from build123d import *

# Parameters (mm, degrees)
IZIM1_W                     = 30
IZIM1_H                     = 30
IZIM1_R                     = 4.75
Y_KSEKLIK_EKSTR_ZYON1_DEPTH = 5
IZIM2_R                     = 10
IZIM2_R_2                   = 4.75
Y_KSEKLIK_EKSTR_ZYON2_DEPTH = 20
IZIM3_R                     = 1.5
KES_EKSTR_ZYON1_DEPTH       = 7


with BuildPart() as part:
    # Çizim1 → Yükseklik-Ekstrüzyon1 (new body)
    with BuildSketch(Plane(origin=(0, 0, 0), x_dir=(1, 0, 0), z_dir=(0, 1, 0))):
        with Locations((15, 15)):
            Rectangle(IZIM1_W, IZIM1_H)
        with Locations(Location((15, 15, 0), (0, 0, 270))):
            Circle(IZIM1_R, mode=Mode.SUBTRACT)
    extrude(amount=Y_KSEKLIK_EKSTR_ZYON1_DEPTH)

    # Çizim2 → Yükseklik-Ekstrüzyon2 (add)
    with BuildSketch(Plane(origin=(0, 5, 0), x_dir=(1, 0, 0), z_dir=(0, 1, 0))):
        with Locations(Location((15, 15, 0), (0, 0, 90))):
            Circle(IZIM2_R)
        with Locations(Location((15, 15, 0), (0, 0, 270))):
            Circle(IZIM2_R_2, mode=Mode.SUBTRACT)
    extrude(amount=Y_KSEKLIK_EKSTR_ZYON2_DEPTH)

    # Çizim3 → Kes-Ekstrüzyon1 (cut)
    with BuildSketch(Plane(origin=(0, 5, 0), x_dir=(1, 0, 0), z_dir=(0, 1, 0))):
        with Locations(Location((4, 26, 0), (0, 0, 270))):
            Circle(IZIM3_R)
        with Locations(Location((26, 26, 0), (0, 0, 270))):
            Circle(IZIM3_R)
        with Locations(Location((26, 4, 0), (0, 0, 270))):
            Circle(IZIM3_R)
        with Locations(Location((4, 4, 0), (0, 0, 270))):
            Circle(IZIM3_R)
    extrude(amount=-KES_EKSTR_ZYON1_DEPTH, mode=Mode.SUBTRACT)


solid = part.part
Geometry: final body of the model. Coordinates: model frame, mm. A direction names the side the tool comes from. Give positions to 0.01 mm unless a question says otherwise; leave off trailing zeros. Loops run counter-clockwise (first coordinate to the right, second up) from the corner with the lowest first, then second, coordinate; pieces in that order, holes last. Notation, with made-up numbers: (4.25, -20) - (59.25, -20) arc R11 ccw to (59.25, 0) - close; hole circle Ø8 at (48.25, -38.75). An arc over 180 degrees is marked (long way). One line per question, with ' | ' between items. Start each with the question number.
(1) Section query D-D on z = -15.75. Return loops of the section in (x, y).
(2) Ray query, line 1 (X direction, y = 1, z = -26); line 2 (X direction, y = 4.25, z = -3.5); line 3 (X direction, y = 18.5, z = -15). Return the intervals inside material, ascending. Write a range as from..to.
(3) Contact query for flat-ended pins moving along their axis: pin 1 (1.5 mm diameter, centred on y = 14, z = -23.5, fed in from -X); pin 2 (11 mm diameter, centred on x = 15, z = -15, fed in from -Y); pin 3 (3 mm diameter, centred on x = 14.5, y = 10.5, fed in from -Z); pin 4 (8 mm diameter, centred on y = 21.5, z = -14.5, fed in from +X). Output: stop coordinate, or through.
(4) Reachability of faces 1 (the flat face through (11, 0, -19)), 2 (the flat face through (4.8, 5, -15.2)) from +Z, -Z, +X, -X, +Y, -Y: full face, straight path, thin tool, end or side. Return the list, or none.
(5) Section query C-C on x = 15. Return loops of the section in (y, z), then the cut area to 4 significant figures.
(6) Section query A-A on x = 26. Return loops of the section in (y, z).
(7) Section query B-B on z = -26. Return loops of the section in (x, y).
(8) Pull-direction query (Z, two-part tool) for faces 3 (the flat face through (15, 2, 0)), 4 (the flat face through (12.6, 25, -19.3)), 5 (the cylindrical face through (27.487, 2.535, -4.195)); classes: released by +Z, released by -Z, zero draft, split by the parting line, or undercut.
The answers:
1) outline: (0, 0) - (10.31, 0) - (10.31, 25) - (5.03, 25) - (5.03, 5) - (0, 5) - close; (19.69, 0) - (30, 0) - (30, 5) - (24.97, 5) - (24.97, 25) - (19.69, 25) - close
2) line 1: 0..2.5, 5.5..24.5, 27.5..30 | line 2: 0..2.59, 5.41..24.59, 27.41..30 | line 3: 5..10.25, 19.75..25
3) pin 1: x = 8.68 | pin 2: y = 0 | pin 3: z = -25 | pin 4: x = 25
4) face 1: +Z, -Z, +X, -X, -Y | face 2: +Y
5) outline: (0, -30) - (5, -30) - (5, -25) - (25, -25) - (25, -19.75) - (0, -19.75) - close; (0, -10.25) - (25, -10.25) - (25, -5) - (5, -5) - (5, 0) - (0, 0) - close | area: 312.5 mm2
6) outline: (0, -30) - (5, -30) - (5, -27.5) - (0, -27.5) - close; (0, -24.5) - (5, -24.5) - (5, -5.5) - (0, -5.5) - close; (0, -2.5) - (5, -2.5) - (5, 0) - (0, 0) - close
7) outline: (0, 0) - (2.5, 0) - (2.5, 5) - (0, 5) - close; (5.5, 0) - (24.5, 0) - (24.5, 5) - (5.5, 5) - close; (27.5, 0) - (30, 0) - (30, 5) - (27.5, 5) - close
8) face 3: released by +Z | face 4: zero draft | face 5: undercut
